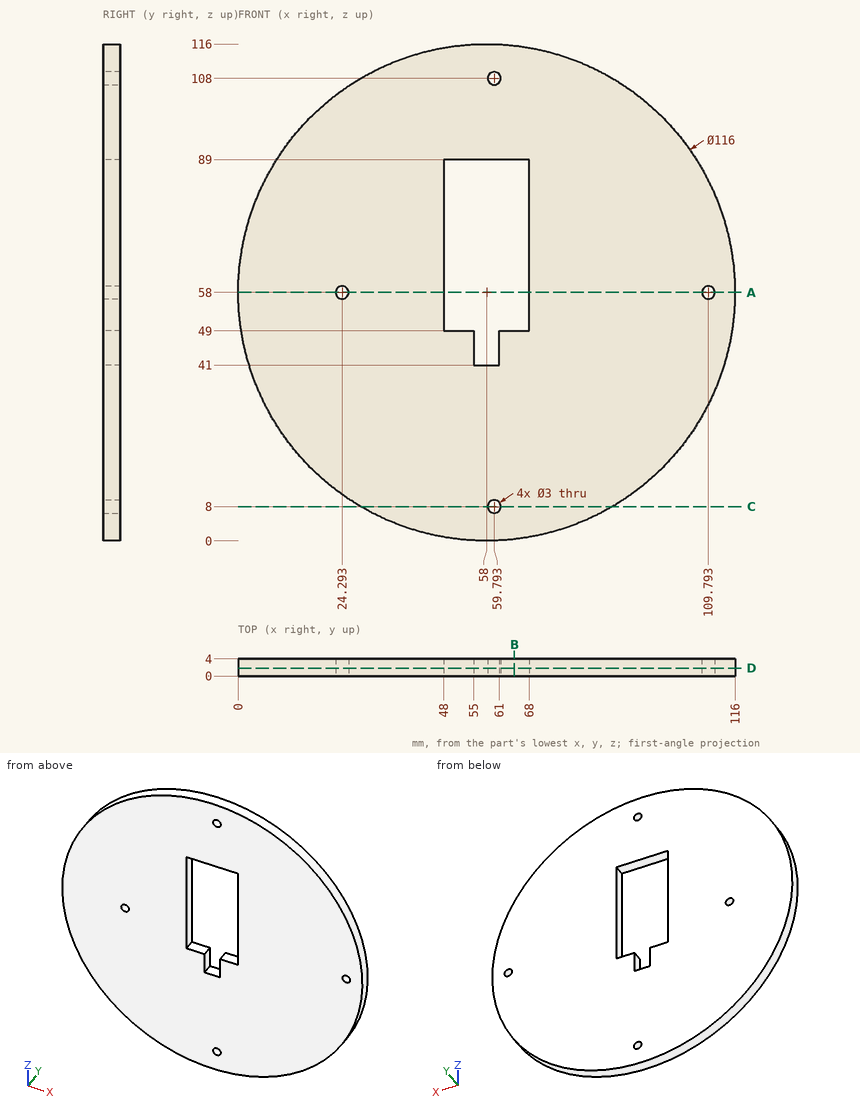
Geometry: see drawing. Coordinates: mm, zero at the bounding-box minimum. Round coordinates to 2 decimals unless told otherwise and drop trailing zeros. Order: outer loops, then holes, each group sorted by start corner. A loop starts at its lowest first (then second) coordinate and runs counter-clockwise, first axis right, second up. Notation, with made-up numbers: (32, -29) -> (65, -29) arc R21 cw to (65, -2) -> close; hole circle Ø11 at (50.5, 34). An arc over 180 degrees is marked (long way). Write each question's results on one line, items separated by ' | '.
Q1. Section query B-B (x = 64.5). Output: boundary loops of the cut face in (y, z) (1 decimal).
Response values:
outline: (0, 0.4) -> (4, 0.4) -> (4, 49) -> (0, 49) -> close; (0, 89) -> (4, 89) -> (4, 115.6) -> (0, 115.6) -> close
Q2. Section query A-A (z = 58). Output: boundary loops of the cut face in (x, y).
Response values:
outline: (0, 0) -> (22.79, 0) -> (22.79, 4) -> (0, 4) -> close; (25.79, 0) -> (48, 0) -> (48, 4) -> (25.79, 4) -> close; (68, 0) -> (108.29, 0) -> (108.29, 4) -> (68, 4) -> close; (111.29, 0) -> (116, 0) -> (116, 4) -> (111.29, 4) -> close
Q3. Pin query (flat end, axial travel): pin 1 Ø1.2 at (y, z) = (1, 47) entering from -X; pin 2 Ø1 at (x, y) = (80.5, 2) entering from +Z (1 decimal); pin 3 Ø1.2 at (x, y) = (60, 1.5) entering from -Z; pin 4 Ø1.8 at (x, z) = (59.79, 8) entering from -Y. Return the tip coordinate at first contact, or that it passes through.
Response values:
pin 1: x = 0.94 | pin 2: z = 111.7 | pin 3: z = 0.02 | pin 4: through
Q4. Ray query, line 1 along X through (y, z) = (1.75, 58); line 2 along X through (y, z) = (2.75, 57) (1 decimal); line 3 along X through (y, z) = (1.7, 108) (1 decimal). Return the intervals inside material, ascending.
Response values:
line 1: 0 to 22.79, 25.79 to 48, 68 to 108.29, 111.29 to 116 | line 2: 0 to 23.2, 25.4 to 48, 68 to 108.7, 110.9 to 116 | line 3: 28.6 to 58.3, 61.3 to 87.4
Q5. Section query D-D (y = 1.85). Output: boundary loops of the cut face in (x, z), and give its area (3 significant figures).
Response values:
outline: circle Ø116 at (58, 58); hole circle Ø3 at (24.29, 58); hole (48, 49) -> (55, 49) -> (55, 41) -> (61, 41) -> (61, 49) -> (68, 49) -> (68, 89) -> (48, 89) -> close; hole circle Ø3 at (59.79, 8); hole circle Ø3 at (59.79, 108); hole circle Ø3 at (109.79, 58) | area: 9,690 mm²
Q6. Section query C-C (z = 8). Output: boundary loops of the cut face in (x, y), and give its area (3 significant figures).
Response values:
outline: (28.61, 0) -> (58.29, 0) -> (58.29, 4) -> (28.61, 4) -> close; (61.29, 0) -> (87.39, 0) -> (87.39, 4) -> (61.29, 4) -> close | area: 223 mm²
